Work out the finished part from the listing and answer in its coordinate system (mm). Face numbers are marked on the shaded views. A direction names the side the tool comes from. Round coordinates to 2 decimals unless told otherwise and drop trailing zeros. Loops run counter-clockwise (first coordinate to the right, second up) from the corner with the lowest first, then second, coordinate; pieces in that order, holes last. Notation, with made-up numbers: (40, 3) -> (56, 3) arc R25 cw to (56, 18) -> close; hole circle Ø11 at (-8.75, 47.25). An arc over 180 degrees is marked (long way). Use one line per item in the form item = value.
```python
from build123d import *

# Parameters (mm, degrees)
SKETCH1_R           = 24
BOSS_EXTRUDE1_DEPTH = 12
SKETCH3_R           = 25.5
BOSS_EXTRUDE3_DEPTH = 1.5
SKETCH4_R           = 25.5
BOSS_EXTRUDE4_DEPTH = 1.5
SKETCH5_R           = 19
BOSS_EXTRUDE5_DEPTH = 10
SKETCH6_R           = 6
CUT_EXTRUDE1_DEPTH  = 25


with BuildPart() as part:
    # Sketch1 → Boss-Extrude1 (new body)
    with BuildSketch(Plane(origin=(0, 0, 0), x_dir=(1, 0, 0), z_dir=(0, 1, 0))):
        Circle(SKETCH1_R)
    extrude(amount=BOSS_EXTRUDE1_DEPTH)

    # Sketch3 → Boss-Extrude3 (add)
    with BuildSketch(Plane(origin=(0, 12, 0), x_dir=(1, 0, 0), z_dir=(0, 1, 0))):
        Circle(SKETCH3_R)
    extrude(amount=BOSS_EXTRUDE3_DEPTH)

    # Sketch4 → Boss-Extrude4 (add)
    with BuildSketch(Plane.XZ):
        Circle(SKETCH4_R)
    extrude(amount=BOSS_EXTRUDE4_DEPTH)

    # Sketch5 → Boss-Extrude5 (add)
    with BuildSketch(Plane.XZ.offset(1.5)):
        Circle(SKETCH5_R)
    extrude(amount=BOSS_EXTRUDE5_DEPTH)

    # Sketch6 → Cut-Extrude1 (cut)
    with BuildSketch(Plane(origin=(0, 13.5, 0), x_dir=(1, 0, 0), z_dir=(0, 1, 0))):
        Circle(SKETCH6_R)
    extrude(amount=-CUT_EXTRUDE1_DEPTH, mode=Mode.SUBTRACT)


solid = part.part
```
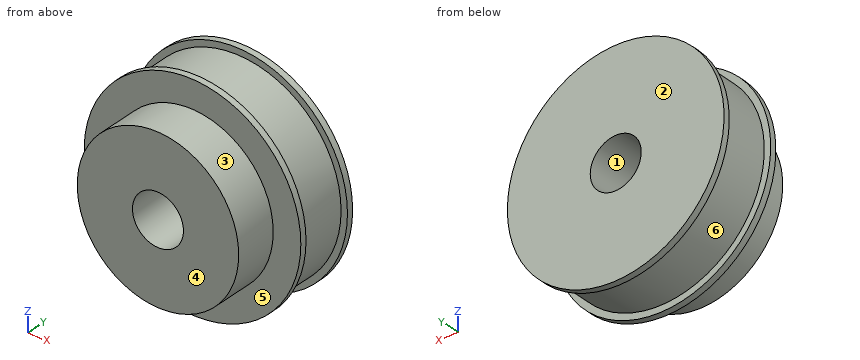
(1) Find section D-D, the plane x = 20.5. Write down the section's boundary in (y, z), then the cut area to 3 significant figures.
Completed:
outline = (-1.5, -15.17) -> (0, -15.17) -> (0, -12.48) -> (12, -12.48) -> (12, -15.17) -> (13.5, -15.17) -> (13.5, 15.17) -> (12, 15.17) -> (12, 12.48) -> (0, 12.48) -> (0, 15.17) -> (-1.5, 15.17) -> close
area = 391 mm2
(2) Find section B-B, the plane x = 0. Write down the section's boundary in (y, z).
Completed:
outline = (-11.5, -19) -> (-1.5, -19) -> (-1.5, -25.5) -> (0, -25.5) -> (0, -24) -> (12, -24) -> (12, -25.5) -> (13.5, -25.5) -> (13.5, -6) -> (-11.5, -6) -> close; (-11.5, 6) -> (13.5, 6) -> (13.5, 25.5) -> (12, 25.5) -> (12, 24) -> (0, 24) -> (0, 25.5) -> (-1.5, 25.5) -> (-1.5, 19) -> (-11.5, 19) -> close
(3) Given P1, Ø3, axis at y = 0, z = -18.5, coming from the -X side; P2, Ø8, axis at x = -15.5, y = 5.5, coming from the +Z side; P3, Ø3, axis at y = 7, z = -17, coming from the +X side, each flat-ended and moving along its own axis, determine where each tip first touches the part or whether it passes through.
Completed:
P1 = -19.01
P2 = 21.07
P3 = 18.32
(4) Consider L1, parallel to Z at x = 0, y = 7; L2, parallel to Z at x = 0, y = -0.75. Determine where each line is inside the solid, lowest interval first.
Completed:
L1 = -24 to -6, 6 to 24
L2 = -25.5 to -6, 6 to 25.5
(5) Find section C-C, the plane y = -4. Write down the section's boundary in (x, z).
Completed:
outline = circle Ø38 at (0, 0); hole circle Ø12 at (0, 0)
(6) For a pull along X with two mould halves and no side action, classify the marked faces 1, 2 and 3 as +X half, -X half, draft (parallel to the pull), parting line (faces both ways), or undercut.
Completed:
face_1 = undercut
face_2 = draft
face_3 = parting line
(7) For the marked faces 4, 5 and 6, determine the directions among +Z, -Z, +X, -X, +Y, -Y from which every point of the face is accessible in a straight line to the end or side of a thin tool.
Completed:
face_4 = +Z, -Z, +X, -X, -Y
face_5 = -Y
face_6 = none
(8) Find section A-A, the plane z = 0. Write down the section's boundary in (x, y), then the cut area to 3 significant figures.
Completed:
outline = (-25.5, -1.5) -> (-19, -1.5) -> (-19, -11.5) -> (-6, -11.5) -> (-6, 13.5) -> (-25.5, 13.5) -> (-25.5, 12) -> (-24, 12) -> (-24, 0) -> (-25.5, 0) -> close; (6, -11.5) -> (19, -11.5) -> (19, -1.5) -> (25.5, -1.5) -> (25.5, 0) -> (24, 0) -> (24, 12) -> (25.5, 12) -> (25.5, 13.5) -> (6, 13.5) -> close
area = 809 mm2
